Check sheet for the drawn part. Datum: minimum x, y, z corner. Units: mm. A direction names the side the tool comes from. Round coordinates to 2 decimals unless told otherwise and drop trailing zeros. Write each loop counter-clockwise with the first axis right and the second up, starting at its lowest first coordinate (ties: lowest second). Pieces come first, ordered by that corner, then holes. Notation, with made-up numbers: M 14,-27.5 L 55,-27.5 A20 cw 55,0.5 Z; hole C 66,67 d1. An arc over 180 degrees is marked long. Put each result on its own line as item: value.
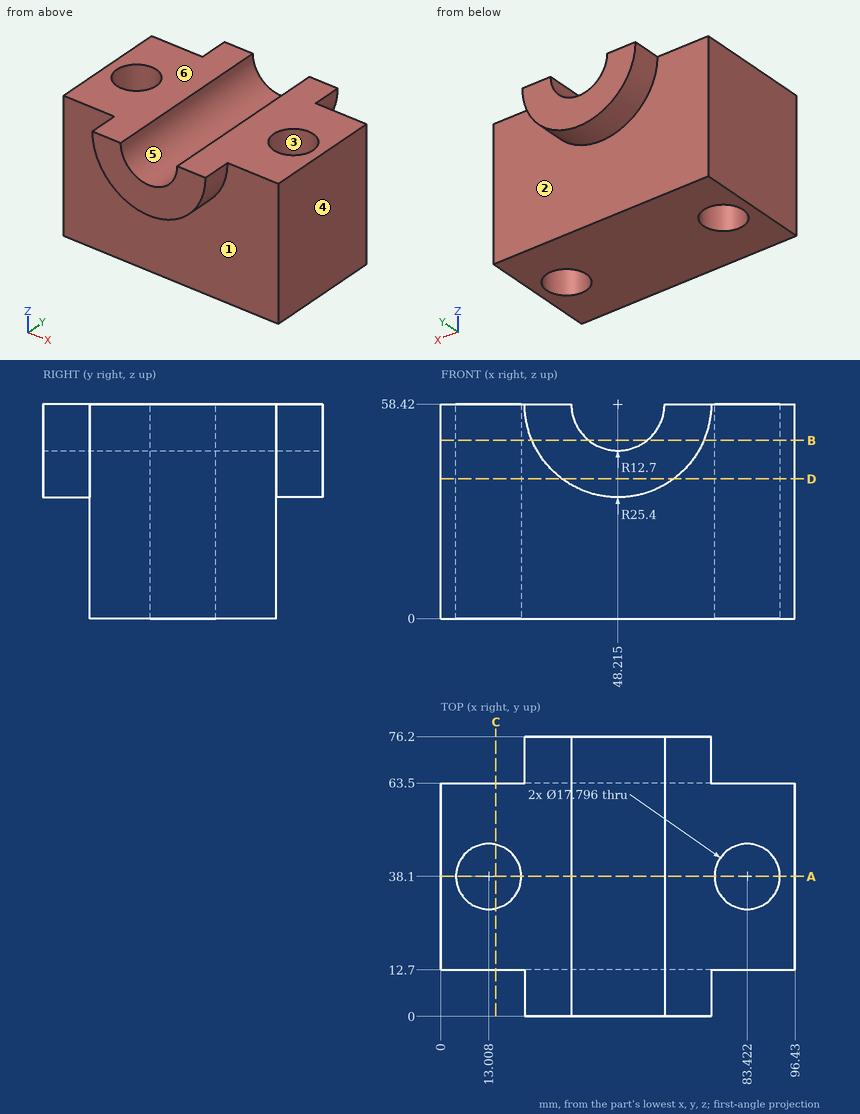
1. Scan lines: probe 1 along X at (y, z) = (38, 21) (1 decimal); probe 2 along Y at (x, z) = (83, 18.5); probe 3 along X at (y, z) = (39.5, 3) (1 decimal). Record each from-to range of solid material in increasing order.
Computed values:
probe 1: x = 0 to 4.1, 21.9 to 74.5, 92.3 to 96.4
probe 2: y = 12.7 to 29.21, 46.99 to 63.5
probe 3: x = 0 to 4.2, 21.8 to 74.6, 92.2 to 96.4
2. Cross-section at B-B (z = 48.5). Enter the section's corners in (x, y) (1 decimal).
Computed values:
outline: M 0,12.7 L 24.8,12.7 L 24.8,0 L 40.3,0 L 40.3,76.2 L 24.8,76.2 L 24.8,63.5 L 0,63.5 Z; M 56.1,0 L 71.6,0 L 71.6,12.7 L 96.4,12.7 L 96.4,63.5 L 71.6,63.5 L 71.6,76.2 L 56.1,76.2 Z; hole C 13,38.1 d17.8; hole C 83.4,38.1 d17.8
3. Release check for a two-part mould opening along X. For the marked faces 4, 5 and 6 record: +X half, -X half, draft (parallel to the pull), parting line (faces both ways), or undercut.
Computed values:
face 4: +X half
face 5: undercut
face 6: draft
4. Depth check by flat-ended pin: pin 1 Ø10.5 at (x, y) = (83.42, 38.1) entering from -Z; pin 2 Ø1 at (x, z) = (75.5, 25.5) entering from -Y. Enter the tip coordinate at first touch or a pass-through.
Computed values:
pin 1: passes through
pin 2: stops at y = 12.7
5. Cross-section at A-A (y = 38.1). Enter the section's corners in (x, z) (1 decimal), then the cut area to 3 significant figures.
Computed values:
outline: M 0,0 L 4.1,0 L 4.1,58.4 L 0,58.4 Z; M 21.9,0 L 74.5,0 L 74.5,58.4 L 60.9,58.4 A12.7 cw 35.5,58.4 L 21.9,58.4 Z; M 92.3,0 L 96.4,0 L 96.4,58.4 L 92.3,58.4 Z
area: 3,300 mm2
6. Access from +Z, -Z, +X, -X, +Y, -Y to the whole of each face (thin tool, end or side, straight path). Record for the marked faces 1, 2 and 3.
Computed values:
face 1: -Z, -Y
face 2: -Z, +Y
face 3: +Z, -Z
7. Cross-section at C-C (x = 15). Enter the section's corners in (y, z), then the cut area to 3 significant figures.
Computed values:
outline: M 12.7,0 L 29.43,0 L 29.43,58.42 L 12.7,58.42 Z; M 46.77,0 L 63.5,0 L 63.5,58.42 L 46.77,58.42 Z
area: 1,950 mm2
8. Cross-section at D-D (z = 38). Enter the section's corners in (x, y) (1 decimal).
Computed values:
outline: M 0,12.7 L 33.1,12.7 L 33.1,0 L 63.3,0 L 63.3,12.7 L 96.4,12.7 L 96.4,63.5 L 63.3,63.5 L 63.3,76.2 L 33.1,76.2 L 33.1,63.5 L 0,63.5 Z; hole C 13,38.1 d17.8; hole C 83.4,38.1 d17.8
